Part model, mm, in its own coordinate system. Face numbers are marked on the shaded views. A direction names the side the tool comes from. Round coordinates to 2 decimals unless told otherwise and drop trailing zeros. Loops run counter-clockwise (first coordinate to the right, second up) from the corner with the lowest first, then second, coordinate; pieces in that order, holes last. Notation, with made-up numbers: M 67,0.25 L 122,0.25 A17 cw 122,32.25 Z; hole C 64,16 d11. An arc over 180 degrees is marked long. Write each question's results on one line, items separated by ' | '.
from build123d import *

# Parameters (mm, degrees)
EXTRUDE_1_DEPTH     = 109
EXTRUDE_2_DEPTH     = 18
SKETCH_3_W          = 25
SKETCH_3_H          = 11.25
CUT_EXTRUDE_1_DEPTH = 18
SKETCH_4_W          = 25
SKETCH_4_H          = 27
EXTRUDE_3_DEPTH     = 27
CUT_EXTRUDE_2_DEPTH = 122.166018853
CUT_EXTRUDE_3_DEPTH = 166.462013552
FILLET_1_R          = 3


# Read off the part's stored shape, not the designer's step: Бобышка-Вытянуть2
with BuildPart() as part:
    # Эскиз1 → Бобышка-Вытянуть1 (new, symmetric)
    with BuildSketch(Plane(origin=(0, 0, 0), x_dir=(0, 0, -1), z_dir=(1, 0, 0))):
        with BuildLine():
            Line((11, 0), (25.25, 0))
            Line((25.25, 0), (25.25, -9))
            Line((25.25, -9), (-25.25, -9))
            Line((-25.25, -9), (-25.25, 0))
            Line((-25.25, 0), (-11, 0))
            ThreePointArc((-11, 0), (0, 6), (11, 0))
        make_face()
    extrude(amount=EXTRUDE_1_DEPTH, both=True)

    # Бобышка-Вытянуть2 outline → Бобышка-Вытянуть2 (add)
    with BuildSketch(Plane(origin=(0, 0, 0), x_dir=(1, 0, 0), z_dir=(0, 1, 0))):
        Polygon((16, 11), (20.656976684, -11), (29.856406461, -11), (25.199429777, 11), align=None)
        Polygon((-29.856406461, -11), (-20.656976684, -11), (-16, 11), (-25.199429777, 11), align=None)
        Polygon((78.012123179, -10.999996132), (86.400679256, -10.994643711), (93.506557878, -2.272856192), (100.623560797, -10.985568626), (109.012116871, -10.980216204), (93.499996845, 8.009889964), align=None)
        Polygon((64.623554487, -11.008538874), (73.012110561, -11.003186452), (57.499990534, 7.986919716), (42.012116871, -11.02296638), (50.400672946, -11.017613959), (57.506551567, -2.29582644), align=None)
        Polygon((-109.012116871, -10.980216204), (-100.623560797, -10.985568626), (-93.506557878, -2.272856192), (-86.400679256, -10.994643711), (-78.012123179, -10.999996132), (-93.499996845, 8.009889964), align=None)
        Polygon((-73.012110561, -11.003186452), (-64.623554487, -11.008538874), (-57.506551567, -2.29582644), (-50.400672946, -11.017613959), (-42.012116871, -11.02296638), (-57.499990534, 7.986919716), align=None)
    extrude(amount=EXTRUDE_2_DEPTH)

    # Эскиз3 → Вырез-Вытянуть1 (cut)
    with BuildSketch(Plane(origin=(0, 0, 0), x_dir=(1, 0, 0), z_dir=(0, 1, 0))):
        with Locations((0, 19.625)):
            Rectangle(SKETCH_3_W, SKETCH_3_H)
        with Locations((0, -19.625)):
            Rectangle(SKETCH_3_W, SKETCH_3_H)
    extrude(amount=-CUT_EXTRUDE_1_DEPTH, mode=Mode.SUBTRACT)

    # Эскиз4 → Бобышка-Вытянуть3 (add)
    with BuildSketch(Plane.XZ.offset(9)):
        with Locations((38, 0)):
            Rectangle(SKETCH_4_W, SKETCH_4_H)
        with Locations((-38, 0)):
            Rectangle(SKETCH_4_W, SKETCH_4_H)
    extrude(amount=EXTRUDE_3_DEPTH)

    # Эскиз6 → Вырез-Вытянуть2 (cut, through all)
    with BuildSketch(Plane.XY.offset(13.5)):
        Polygon((-50.5, -9), (-50.5, -36), (-44.5, -36), align=None)
        Polygon((-25.5, -36), (-31.5, -36), (-25.5, -9), align=None)
        Polygon((25.5, -9), (25.5, -36), (31.5, -36), align=None)
        Polygon((50.5, -36), (44.5, -36), (50.5, -9), align=None)
    extrude(amount=-CUT_EXTRUDE_2_DEPTH, mode=Mode.SUBTRACT)

    # Эскиз5 → Вырез-Вытянуть3 (cut, through all)
    with BuildSketch(Plane.ZY.offset(50.5)):
        Polygon((-13.5, -9), (-13.5, -36), (-6.5, -36), align=None)
        Polygon((13.5, -36), (6.5, -36), (13.5, -9), align=None)
    extrude(amount=-CUT_EXTRUDE_3_DEPTH, mode=Mode.SUBTRACT)

    # Скругление1
    fillet_1_edges = [part.edges().sort_by_distance(p)[0] for p in [
        (-38, -36, -6.5),
        (38, -36, -6.5),
        (-38, -36, 6.5),
        (38, -36, 6.5),
    ]]
    fillet(fillet_1_edges, radius=FILLET_1_R)


solid = part.part
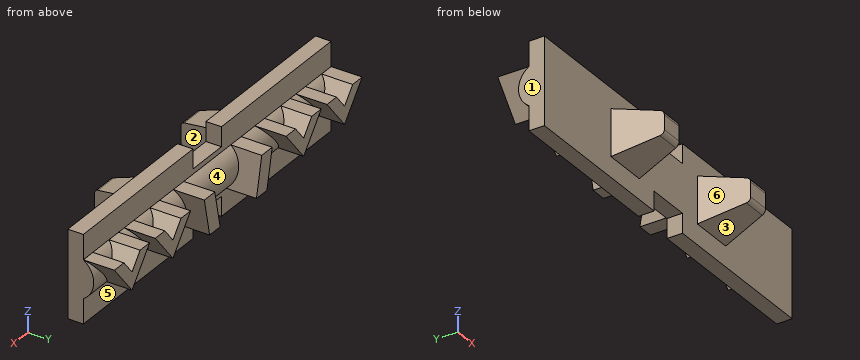
Item 1: Wall check: L1, parallel to X at y = 11, z = 0; L2, parallel to X at y = 9.5, z = 1; L3, parallel to Y at x = 90.5, z = -12. Give the ranges that are in metal, low to high.
Filled sheet:
L1: -100.04 to -86.97, -64.02 to -50.99, -27.53 to -18.33, 18.33 to 27.53, 50.99 to 64.02, 86.97 to 100.04 | L2: -100.86 to -86.16, -64.84 to -50.18, -27.74 to -18.54, 18.54 to 27.74, 50.18 to 64.84, 86.16 to 100.86 | L3: -9 to 0
Item 2: Band-saw the part on B-B on y = -16. Give the cut face in (x, z).
Filled sheet:
outline: M -48.94,-11.69 L -27.06,-11.69 L -27.06,11.69 L -48.94,11.69 Z; M 27.06,-11.69 L 48.94,-11.69 L 48.94,11.69 L 27.06,11.69 Z
Item 3: Which spindle directions (+Z, -Z, +X, -X, +Y, -Y) get a long thin tool onto all of the face, cutting with end or side? Do the marked faces 4, 5 and 6. Say none if no direction does.
Filled sheet:
face 4: +Y | face 5: -Z, +X, -X, +Y | face 6: +Z, -Z, -Y
Item 4: Band-saw the part on A-A on z = -21. Give the cut face in (x, y), and give its area (3 significant figures).
Filled sheet:
outline: M -109,-9 L -12.5,-9 L -12.5,0 L -109,0 Z; M 12.5,-9 L 109,-9 L 109,0 L 12.5,0 Z | area: 1,740 mm^2
Item 5: Drop flat-ended pins along their axis: P1, Ø10, axis at y = -3, z = 21, coming from the +X side; P2, Ø4.5, axis at x = -12, z = 18.5, coming from the +Y side; P3, Ø7.5, axis at x = 24.5, y = 7.5, coming from the +Z side; P4, Ø6, axis at x = 72, y = -13, coming from the -Z side. Give the stop position or say it passes through.
Filled sheet:
P1: x = 109 | P2: y = 0 | P3: z = 11 | P4: through
Item 6: Band-saw the part on C-C on y = -2. Give the cut face in (x, z).
Filled sheet:
outline: M -109,-25.25 L -12.5,-25.25 L -12.5,-14 L 12.5,-14 L 12.5,-25.25 L 109,-25.25 L 109,25.25 L 12.5,25.25 L 12.5,14 L -12.5,14 L -12.5,25.25 L -109,25.25 Z
Item 7: Two-plate mould, pull along X, no slides. Class the marked faces 1, 2 and 3: +X half, -X half, draft (parallel to the pull), parting line (faces both ways), or undercut.
Filled sheet:
face 1: -X half | face 2: undercut | face 3: draft
